Here's the drawing with two shaded views (mm, measured from the low corner). I have some questions. A direction names the side the tool comes from. Give positions to 0.01 mm unless a question says otherwise; leave off trailing zeros. Loops run counter-clockwise (first coordinate to the right, second up) from the corner with the lowest first, then second, coordinate; pieces in that order, holes last. Notation, with made-up numbers: M 56.5,53.25 L 94.5,53.25 A29 cw 94.5,86.25 Z; hole C -16,-25 d9. An arc over 180 degrees is marked long. Write item = value, one per line. Start each with the question number.
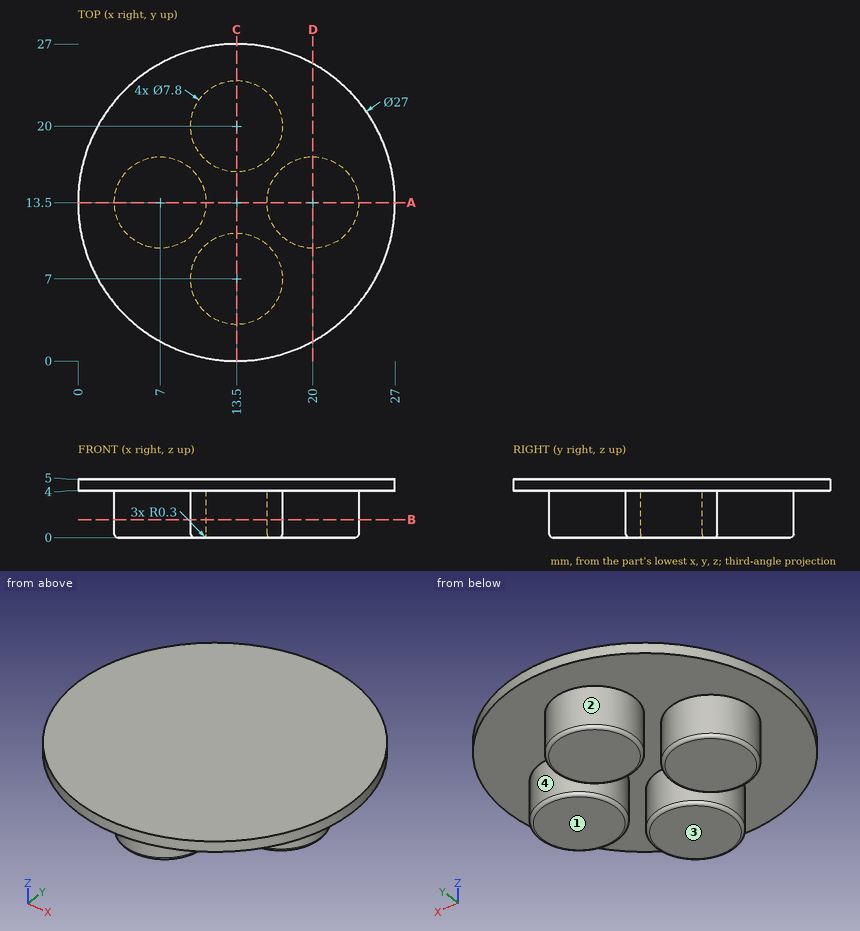
Q1. If we section it at A-A, the plane y = 13.5: List the corners of the cut face in (x, z) for me, then the cut area to 3 significant figures.
Q2. If I drill on line 1 along Y through (x, z) = (13.25, 1.6); line 2 along Y through (x, z) = (10.5, 2.5), over which ranges is the centre line in solid material (lowest first)?
Q3. On a 3-axis mill with a long thin cutter (end or side, diameter ignored), from which of +Z, -Z, +X, -X, +Y, -Y can I reach the whole of each face in a straight line? I mean the marked faces 3 and 4. Say none if no direction works.
Q4. Will these pins go through, and if not, where does the flat tip stop? pin 1 (1 mm diameter, centred on y = 13.5, z = 2, fed in from -X); pin 2 (1 mm diameter, centred on x = 12.5, z = 1, fed in from +Y).
Q5. If we section it at D-D, the plane x = 20: List the corners of the cut face in (y, z) for me.
Q6. We'd pull the mould along Y, two halves only. Please class the marked faces 1 and 2: pulls with the +Y half, pulls with the -Y half, needs draft (parallel to the pull), parting line crosses it, or undercut.
Q7. If we section it at B-B, the plane z = 1.55: List the corners of the cut face in (x, y) for me.
Resolved:
q1.outline = M 0,4 L 3.1,4 L 3.1,0.3 A0.3 ccw 3.4,0 L 10.6,0 A0.3 ccw 10.9,0.3 L 10.9,4 L 16.1,4 L 16.1,0.3 A0.3 ccw 16.4,0 L 23.6,0 A0.3 ccw 23.9,0.3 L 23.9,4 L 27,4 L 27,5 L 0,5 Z
q1.area = 89.3 mm²
q2.line_1 = 3.11 to 10.89, 16.11 to 23.89
q2.line_2 = 4.51 to 9.49, 11.78 to 15.22, 17.51 to 22.49
q3.face_3 = -Z, +X, -X, +Y, -Y
q3.face_4 = -Z
q4.pin_1 = 3.1
q4.pin_2 = 23.87
q5.outline = M 1.67,4 L 9.6,4 L 9.6,0.3 A0.3 ccw 9.9,0 L 17.1,0 A0.3 ccw 17.4,0.3 L 17.4,4 L 25.33,4 L 25.33,5 L 1.67,5 Z
q6.face_1 = needs draft
q6.face_2 = undercut
q7.outline = C 7,13.5 d7.8; C 13.5,7 d7.8; C 13.5,20 d7.8; C 20,13.5 d7.8
